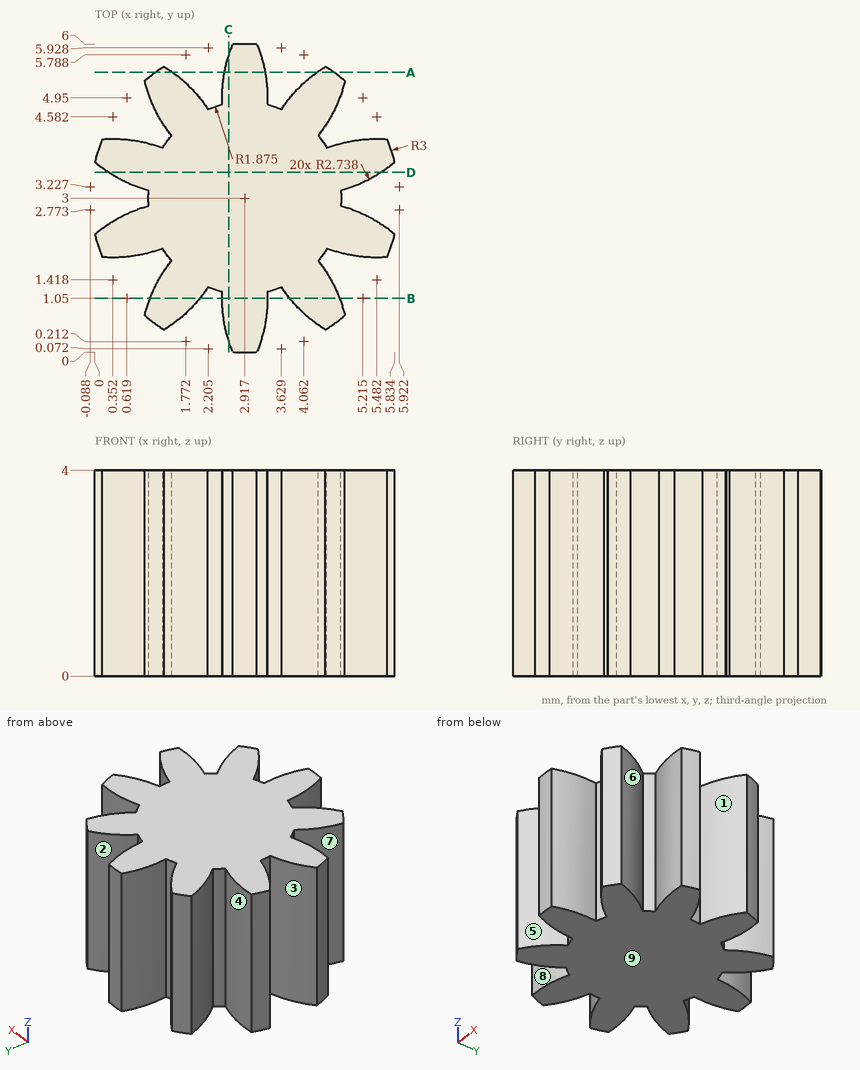
Drawing for the job (mm, zero at the part's lowest x, y, z). A direction names the side the tool comes from. Round coordinates to 2 decimals unless told otherwise and drop trailing zeros. Loops run counter-clockwise (first coordinate to the right, second up) from the corner with the lowest first, then second, coordinate; pieces in that order, holes last. Notation, with made-up numbers: (-2.5, 41) -> (5.5, 41) arc R19 ccw to (5.5, 49) -> close; hole circle Ø5 at (43, 18.5). An arc over 180 degrees is marked (long way). Answer in a Markdown table with one row per item.
Item 1: Saw through at C-C (x = 2.6). Write the cut outline in (y, z).
Answers below:
| item | result |
|---|---|
| outline | (0.24, 0) -> (5.76, 0) -> (5.76, 4) -> (0.24, 4) -> close |
Item 2: Mould opens along X. For the marked faces 6, 7, 8 and 9 say: +X half, -X half, draft (parallel to the pull), parting line (faces both ways), or undercut.
Answers below:
| item | result |
|---|---|
| face 6 | +X half |
| face 7 | -X half |
| face 8 | undercut |
| face 9 | draft |
Item 3: Saw through at B-B (y = 1.05). Write the cut outline in (x, z).
Answers below:
| item | result |
|---|---|
| outline | (1.07, 0) -> (2.04, 0) -> (2.04, 4) -> (1.07, 4) -> close; (2.48, 0) -> (3.36, 0) -> (3.36, 4) -> (2.48, 4) -> close; (3.79, 0) -> (4.76, 0) -> (4.76, 4) -> (3.79, 4) -> close |
Item 4: Drill centre lines: L1, parallel to X at y = 0.6, z = 0.65 (1 decimal); L2, parallel to X at y = 5.05, z = 0.5 (1 decimal); L3, parallel to Y at x = 0.55, z = 0.4. Where is each one in solid material? Low to high. Write a range as [from, to].
Answers below:
| item | result |
|---|---|
| L1 | x = [1.1, 1.6], [2.5, 3.3], [4.3, 4.7] |
| L2 | x = [1, 2], [2.5, 3.4], [3.9, 4.8] |
| L3 | y = [1.85, 2.66], [3.34, 4.15] |
Item 5: Saw through at D-D (y = 3.5). Write the cut outline in (x, z).
Answers below:
| item | result |
|---|---|
| outline | (0.27, 0) -> (5.57, 0) -> (5.57, 4) -> (0.27, 4) -> close |
Item 6: Pin check, flat tips, straight feed: pin 1 (3 mm diameter, centred on x = 2.5, y = 4.5, fed in from -Z); pin 2 (2 mm diameter, centred on x = 1, z = 2.5, fed in from -Y); pin 3 (1.5 mm diameter, centred on y = 5, z = 2, fed in from -X). Stop position of each tip, or through.
Answers below:
| item | result |
|---|---|
| pin 1 | stops at z = 0 |
| pin 2 | stops at y = 0.44 |
| pin 3 | stops at x = 0.97 |
Item 7: Saw through at A-A (y = 5.45). State how many separate pieces and enclosed holes the cut face has.
Answers below:
| item | result |
|---|---|
| separate pieces | 3 |
| enclosed holes | 0 |
Item 8: Which spindle directions (+Z, -Z, +X, -X, +Y, -Y) get a long thin tool onto all of the face, cutting with end or side? Do the marked faces 1, 2, 3, 4 and 5. Say none if no direction does.
Answers below:
| item | result |
|---|---|
| face 1 | +Z, -Z, +X |
| face 2 | +Z, -Z, +Y |
| face 3 | +Z, -Z, -X |
| face 4 | +Z, -Z |
| face 5 | +Z, -Z, -Y |
